Input: part model. Units: mm. Frame: model coordinates. Coordinates: 2 decimals unless noted, no trailing zeros. Write each loop counter-clockwise with the first axis right and the second up, starting at its lowest first coordinate (ties: lowest second). Pieces come first, ordered by that corner, then holes. Notation, with made-up numbers: M 3,27.25 L 28,27.25 A16 ccw 28,50.25 Z; hole C -22,-12.75 d5. An arc over 180 degrees is marked long. Write each question's results on one line, items separated by ' | '. Start each with the question number.
1. First-contact query: pin 1 (1.8 mm diameter, centred on y = 23, z = 91.5, fed in from +X); pin 2 (4 mm diameter, centred on y = -11, z = 249, fed in from +X); pin 3 (1 mm diameter, centred on x = -20.5, y = -15, fed in from -Z); pin 4 (1 mm diameter, centred on y = 1.5, z = 190, fed in from -X). Flat tips, straight axial feed; report the tip coordinate or a pass-through.
2. Pull-direction query (Z, two-part tool) for faces 1 (the cylindrical face through (0.1, 21.5, 92.7)), 2 (the flat face through (0, 0, 300)), 3 (the flat face through (0, 0, 0)); classes: +Z half, -Z half, draft (parallel to the pull), parting line (faces both ways), or undercut.
3. Ray query, probe 1 along X at (y, z) = (1, 287); probe 2 along X at (y, z) = (-15.5, 31.5); probe 3 along Y at (x, z) = (-5, 129). Return the intervals inside material, ascending.
4. Section query B-B, the plane y = -8. Output: boundary loops of the cut face in (x, z), and give its area (3 significant figures).
5. Section query C-C, the plane z = 209. Output: boundary loops of the cut face in (x, y), and give its area (3 significant figures).
6. Section query A-A, the plane x = 12. Output: boundary loops of the cut face in (y, z), and give its area (3 significant figures).
```python
from build123d import *

# Parameters (mm, degrees)
SKETCH1_R            = 27.5
BOSS_EXTRUDE1_DEPTH  = 300
CUT_EXTRUDE1_START   = 21.500000052
CUT_EXTRUDE1_DEPTH   = 7.499999948
CUT_EXTRUDE1_START_2 = 20.310644134
CUT_EXTRUDE1_2_DEPTH = 1.189355918
CUT_EXTRUDE1_START_3 = 72.999999946
CUT_EXTRUDE1_3_DEPTH = 40.000000108


with BuildPart() as part:
    # Sketch1 → Boss-Extrude1 (new body)
    with BuildSketch(Plane.XY):
        Circle(SKETCH1_R)
    extrude(amount=BOSS_EXTRUDE1_DEPTH)

    # Cut-Extrude1: read off the stored shape, not the designer's step
    # Cut-Extrude1 outline → Cut-Extrude1 (cut)
    with BuildSketch(Plane(origin=(0, 0, 0), x_dir=(1, 0, 0), z_dir=(0, 1, 0)).offset(CUT_EXTRUDE1_START)):
        with BuildLine():
            Line((-8, -81), (-8, -105))
            add(Edge.make_bspline(
                [(-8, -105), (-8, -106.063035006), (-7.788701178, -107.105523906), (-6.984119374, -109.039699683), (-6.390533847, -109.923095258), (-4.923786882, -111.390000979), (-4.036294094, -111.985161837), (-2.113824822, -112.785621396), (-1.057490709, -112.998980405), (1.04200741, -113.001012103), (2.09275073, -112.792846435), (4.037391687, -111.986238583), (4.915900837, -111.397309074), (7.133041074, -109.181662675), (8, -107.126189888), (8, -105)],
                knots=[0, 0, 0, 0, 0.125, 0.125, 0.25, 0.25, 0.375, 0.375, 0.5, 0.5, 0.625, 0.625, 0.75, 0.75, 1, 1, 1, 1], degree=3))
            Line((8, -105), (8, -81))
            add(Edge.make_bspline(
                [(8, -81), (8, -79.936964994), (7.788701178, -78.894476094), (6.984119374, -76.960300317), (6.390533847, -76.076904742), (4.923786882, -74.609999021), (4.036294094, -74.014838163), (2.113824822, -73.214378604), (1.057490709, -73.001019595), (-1.04200741, -72.998987897), (-2.09275073, -73.207153565), (-4.037391687, -74.013761417), (-4.915900837, -74.602690926), (-7.133041074, -76.818337325), (-8, -78.873810112), (-8, -81)],
                knots=[0, 0, 0, 0, 0.125, 0.125, 0.25, 0.25, 0.375, 0.375, 0.5, 0.5, 0.625, 0.625, 0.75, 0.75, 1, 1, 1, 1], degree=3))
        make_face()
    extrude(amount=CUT_EXTRUDE1_DEPTH, mode=Mode.SUBTRACT)

    # Cut-Extrude1 2 outline → Cut-Extrude1 2 (cut)
    with BuildSketch(Plane(origin=(0, 0, 0), x_dir=(1, 0, 0), z_dir=(0, 1, 0)).offset(CUT_EXTRUDE1_START_2)):
        with BuildLine():
            Line((-8, -81), (-8, -105))
            add(Edge.make_bspline(
                [(-8, -105), (-8, -106.063035006), (-7.788701178, -107.105523906), (-6.984119374, -109.039699683), (-6.390533847, -109.923095258), (-4.923786882, -111.390000979), (-4.036294094, -111.985161837), (-2.113824822, -112.785621396), (-1.057490709, -112.998980405), (1.04200741, -113.001012103), (2.09275073, -112.792846435), (4.037391687, -111.986238583), (4.915900837, -111.397309074), (7.133041074, -109.181662675), (8, -107.126189888), (8, -105)],
                knots=[0, 0, 0, 0, 0.125, 0.125, 0.25, 0.25, 0.375, 0.375, 0.5, 0.5, 0.625, 0.625, 0.75, 0.75, 1, 1, 1, 1], degree=3))
            Line((8, -105), (8, -81))
            add(Edge.make_bspline(
                [(8, -81), (8, -79.936964994), (7.788701178, -78.894476094), (6.984119374, -76.960300317), (6.390533847, -76.076904742), (4.923786882, -74.609999021), (4.036294094, -74.014838163), (2.113824822, -73.214378604), (1.057490709, -73.001019595), (-1.04200741, -72.998987897), (-2.09275073, -73.207153565), (-4.037391687, -74.013761417), (-4.915900837, -74.602690926), (-7.133041074, -76.818337325), (-8, -78.873810112), (-8, -81)],
                knots=[0, 0, 0, 0, 0.125, 0.125, 0.25, 0.25, 0.375, 0.375, 0.5, 0.5, 0.625, 0.625, 0.75, 0.75, 1, 1, 1, 1], degree=3))
        make_face()
    extrude(amount=CUT_EXTRUDE1_2_DEPTH, mode=Mode.SUBTRACT)

    # Cut-Extrude1 3 outline → Cut-Extrude1 3 (add)
    with BuildSketch(Plane.XY.offset(CUT_EXTRUDE1_START_3)):
        with BuildLine():
            ThreePointArc((8, 20.310644234), (0, 21.5), (-8, 20.310644234))
            Line((-8, 20.310644234), (8, 20.310644234))
        make_face()
    extrude(amount=CUT_EXTRUDE1_3_DEPTH)


solid = part.part
```
Answer:
1) pin 1: x = 16.37 | pin 2: x = 25.99 | pin 3: z = 0 | pin 4: x = -27.48
2) face 1: undercut | face 2: +Z half | face 3: -Z half
3) probe 1: -27.48 to 27.48 | probe 2: -22.72 to 22.72 | probe 3: -27.04 to 27.04
4) outline: M -26.31,0 L 26.31,0 L 26.31,300 L -26.31,300 Z | area: 15,800 mm^2
5) outline: C 0,0 d55 | area: 2,380 mm^2
6) outline: M -24.74,0 L 24.74,0 L 24.74,300 L -24.74,300 Z | area: 14,800 mm^2
